Read the model definition and answer for the solid it produces. Units are mm, in the model's axes. A direction names the side the tool comes from. Coordinates: 2 decimals unless noted, no trailing zeros. Order: outer loops, then holes, each group sorted by start corner. A loop starts at its lowest first (then second) coordinate and runs counter-clockwise, first axis right, second up. Notation, with made-up numbers: (53, -18) -> (72, -18) arc R14 cw to (72, -8) -> close; hole circle Ø2 at (4, 17.5). An arc over 180 degrees is marked (long way). Answer as a JSON object with one key per item and string values. Group by question number.
1) Section C-C on z = -6.25 is taken. Determine the outline of the cut face in (x, y).
2) Given pin 1 (1.3 mm diameter, centred on y = 10, z = 2.5, fed in from -X); pin 2 (1.5 mm diameter, centred on x = 44.5, y = 8.5, fed in from +Z); pin 3 (0.9 mm diameter, centred on x = 24.5, z = 2, fed in from +Y); pin 4 (3.5 mm diameter, centred on x = 45, z = 3, fed in from +Y), each flat-ended and moving along its own axis, determine where each tip first touches the part or whether it passes through.
3) Determine the mould class of faces 1 (the flat face through (11, 11.85, 4)), 2 (the flat face through (21, 1, -8.5)), 3 (the flat face through (-6.5, 10, 4)) for opening direction X: released by +X, released by -X, zero draft, split by the parting line, or undercut.
4) A tool of negligible diameter and unlimited length cuts with its end or side. For faces 4 (the flat face through (21, 2.5, 2)), 5 (the flat face through (39.5, 8, 3)), 6 (the flat face through (44, 8, 5.55)), from which of +Z, -Z, +X, -X, +Y, -Y can it reach the whole face along a straight path? Write none if from no direction.
5) Section B-B on y = 13.5 is taken. Determine the outline of the cut face in (x, z), and give its area (3 significant figures).
6) Consider L1, parallel to X at y = 10.5, z = 3; L2, parallel to Y at x = 11, z = 2.5; L3, parallel to Y at x = 19.5, z = -4.25. Determine where each line is inside the solid, lowest interval first.
7) Section D-D on x = 31 is taken. Determine the outline of the cut face in (y, z), and give its area (3 significant figures).
8) Section A-A on x = 1 is taken. Determine the outline of the cut face in (y, z), and give its area (3 significant figures).
from build123d import *

# Parameters (mm, degrees)
F0_W      = 42
F0_H      = 19.35
F1_DEPTH  = 1.25
F2_W      = 2.5
F2_H      = 8.5
F2_H_2    = 1.75
F3_DEPTH  = 42
F4_W      = 2.5
F4_H      = 5
F4_W_2    = 6.75
F4_W_3    = 6.5
F4_H_2    = 10
F5_DEPTH  = 4.3
F6_W      = 5
F6_H      = 1.9
F7_DEPTH  = 6.75
F8_W      = 10
F8_H      = 1.8
F9_DEPTH  = 6.5
F4_W_4    = 6.85
F4_H_3    = 6.95
F10_DEPTH = 5.35
F4_W_5    = 7.5
F4_H_4    = 10.15
F11_DEPTH = 2.65


with BuildPart() as f1:
    # F0 (on Top) → F1 (new body)
    with BuildSketch(Plane.XY):
        with Locations((21, 9.675)):
            Rectangle(F0_W, F0_H)
    extrude(amount=F1_DEPTH)

    # F2 (on face) → F3 (join)
    with BuildSketch(Plane.YZ.offset(42)):
        with Locations((1.25, -4.25)):
            Rectangle(F2_W, F2_H)
        with Locations((1.25, 2.125)):
            Rectangle(F2_W, F2_H_2)
    extrude(amount=-F3_DEPTH)

    # F4 (on face) → F5 (join)
    with BuildSketch(Plane.XY.offset(1.25)):
        with Locations((40.75, 8.35)):
            Rectangle(F4_W, F4_H)
        with Locations((45.375, 8.35)):
            Rectangle(F4_W_2, F4_H)
        with Locations((-3.25, 10)):
            Rectangle(F4_W_3, F4_H_2)
        with Locations((1.25, 10)):
            Rectangle(F4_W, F4_H_2)
    extrude(amount=F5_DEPTH)

    # F6 (on face) → F7 (cut)
    with BuildSketch(Plane.YZ.offset(48.75)):
        with Locations((8.35, 2.2)):
            Rectangle(F6_W, F6_H)
    extrude(amount=-F7_DEPTH, mode=Mode.SUBTRACT)

    # F8 (on face) → F9 (cut)
    with BuildSketch(Plane(origin=(-6.5, 0, 0), x_dir=(0, -1, 0), z_dir=(-1, 0, 0))):
        with Locations((-10, 2.15)):
            Rectangle(F8_W, F8_H)
    extrude(amount=-F9_DEPTH, mode=Mode.SUBTRACT)

    # F4 (on face) → F10 (join)
    with BuildSketch(Plane.XY.offset(1.25)):
        with Locations((10.575, 8.375)):
            Rectangle(F4_W_4, F4_H_3)
    extrude(amount=F10_DEPTH)

    # F4 (on face) → F11 (join)
    with BuildSketch(Plane.XY.offset(1.25)):
        with Locations((22, 8.925)):
            Rectangle(F4_W_5, F4_H_4)
    extrude(amount=F11_DEPTH)


solid = f1.part
Worked answers:
{
 "1": {"outline": "(0, 0) -> (42, 0) -> (42, 2.5) -> (0, 2.5) -> close"},
 "2": {"pin 1": "stops at x = -6.5", "pin 2": "stops at z = 5.55", "pin 3": "stops at y = 14", "pin 4": "stops at y = 10.85"},
 "3": {"face 1": "undercut", "face 2": "zero draft", "face 3": "released by -X"},
 "4": {"face 4": "+Z, +X, -X", "face 5": "+Z, +Y", "face 6": "+Z, +X, +Y, -Y"},
 "5": {"outline": "(-6.5, 3.05) -> (0, 3.05) -> (0, 0) -> (42, 0) -> (42, 1.25) -> (25.75, 1.25) -> (25.75, 3.9) -> (18.25, 3.9) -> (18.25, 1.25) -> (2.5, 1.25) -> (2.5, 5.55) -> (-6.5, 5.55) -> close", "area": "99.4 mm²"},
 "6": {"L1": "x = 0 to 2.5, 7.15 to 14, 18.25 to 25.75, 39.5 to 42", "L2": "y = 0 to 2.5, 4.9 to 11.85", "L3": "y = 0 to 2.5"},
 "7": {"outline": "(0, -8.5) -> (2.5, -8.5) -> (2.5, 0) -> (19.35, 0) -> (19.35, 1.25) -> (2.5, 1.25) -> (2.5, 3) -> (0, 3) -> close", "area": "49.8 mm²"},
 "8": {"outline": "(0, -8.5) -> (2.5, -8.5) -> (2.5, 0) -> (19.35, 0) -> (19.35, 1.25) -> (15, 1.25) -> (15, 5.55) -> (5, 5.55) -> (5, 1.25) -> (2.5, 1.25) -> (2.5, 3) -> (0, 3) -> close", "area": "92.8 mm²"}
}
